Input: part model. Units: mm. Frame: model coordinates. A direction names the side the tool comes from. Coordinates: 2 decimals unless noted, no trailing zeros. Loops run counter-clockwise (first coordinate to the right, second up) from the corner with the lowest first, then second, coordinate; pieces in that order, holes last.
```python
from build123d import *

# Parameters (mm, degrees)
FACE003_W        = 10
FACE003_H        = 3
EXTRUDE003_DEPTH = 1
FACE002_W        = 10
FACE002_H        = 4
EXTRUDE002_DEPTH = 4
FACE001_W        = 8
FACE001_H        = 2.5
EXTRUDE001_DEPTH = 1.5
SKETCH_W         = 15
SKETCH_H         = 17
EXTRUDE_DEPTH    = 10
FACE004_W        = 29
FACE004_H        = 21
EXTRUDE004_DEPTH = 10


with BuildPart() as extrude003:
    # Face003 → Extrude003 (new body)
    with BuildSketch(Plane(origin=(7.5, 21, 2.5), x_dir=(1, 0, 0), z_dir=(0, 1, 0))):
        Rectangle(FACE003_W, FACE003_H)
    extrude(amount=EXTRUDE003_DEPTH)


with BuildPart() as fusion001:
    # Face002 → Extrude002 (new body)
    with BuildSketch(Plane(origin=(7.5, 17, 2), x_dir=(1, 0, 0), z_dir=(0, 1, 0))):
        Rectangle(FACE002_W, FACE002_H)
    extrude(amount=EXTRUDE002_DEPTH)

    # Fusion001: union Extrude003
    add(extrude003.part)


with BuildPart() as extrude001:
    # Face001 → Extrude001 (new body)
    with BuildSketch(Plane(origin=(7.624542, 0, 3.25), x_dir=(1, 0, 0), z_dir=(0, 1, 0))):
        Rectangle(FACE001_W, FACE001_H)
    extrude(amount=-EXTRUDE001_DEPTH)


with BuildPart() as fusion002:
    # Sketch → Extrude (new body)
    with BuildSketch(Plane.XY):
        with Locations((7.5, 8.5)):
            Rectangle(SKETCH_W, SKETCH_H)
    extrude(amount=EXTRUDE_DEPTH)

    # Fusion: union Extrude001
    add(extrude001.part)

    # Fusion002: union Fusion001
    add(fusion001.part)


with BuildPart() as cut:
    # Face004 → Extrude004 (new body)
    with BuildSketch(Plane(origin=(7.5, 10, 0), x_dir=(0, 1, 0), z_dir=(0, 0, 1))):
        Rectangle(FACE004_W, FACE004_H)
    extrude(amount=EXTRUDE004_DEPTH)

    # Cut: cut Fusion002
    add(fusion002.part, mode=Mode.SUBTRACT)


solid = cut.part
```
Item 1: Line query: L1, parallel to Y at x = 13, z = 5; L2, parallel to X at y = 13.5, z = 0.5; L3, parallel to Y at x = 8, z = 3.75. Output: solid intervals per line, ascending.
Result:
L1: y = -4.5 to 0, 17 to 24.5
L2: x = -3 to 0, 15 to 18
L3: y = -4.5 to -1.5, 22 to 24.5
Item 2: Section query A-A (z = 3.5). Output: boundary loops of the cut face in (x, y).
Result:
outline: (-3, -4.5) - (18, -4.5) - (18, 24.5) - (-3, 24.5) - close; hole (0, 0) - (3.62, 0) - (3.62, -1.5) - (11.62, -1.5) - (11.62, 0) - (15, 0) - (15, 17) - (12.5, 17) - (12.5, 22) - (2.5, 22) - (2.5, 17) - (0, 17) - close
Item 3: Mould query, pull axis X, two halves, no side actions, for faces 1 (the face through (7.4, 21.5, 1)), 2 (the face through (17, 10, 0)), 3 (the face through (7, 0, 5)), 4 (the face through (18, 10, 5)). Classes: +X half, -X half, draft (parallel to the pull), parting line (faces both ways), or undercut.
Result:
face 1: undercut
face 2: draft
face 3: undercut
face 4: +X half
Item 4: Reachability of faces 5 (the face through (7, 19, 10)), 6 (the face through (2.5, 19, 2)), 7 (the face through (15, 8, 5)) from +Z, -Z, +X, -X, +Y, -Y: full face, straight path, thin tool, end or side. Return the list, or none.
Result:
face 5: +Z, +X, -X, +Y, -Y
face 6: none
face 7: +Z, -Z
Item 5: Section query B-B (x = 8.25). Output: boundary loops of the cut face in (y, z).
Result:
outline: (-4.5, 0) - (0, 0) - (0, 2) - (-1.5, 2) - (-1.5, 4.5) - (0, 4.5) - (0, 10) - (-4.5, 10) - close; (17, 4) - (22, 4) - (22, 1) - (21, 1) - (21, 0) - (24.5, 0) - (24.5, 10) - (17, 10) - close
Item 6: Section query D-D (y = -0.5). Output: boundary loops of the cut face in (x, z), then the cut area to 3 significant figures.
Result:
outline: (-3, 0) - (18, 0) - (18, 10) - (-3, 10) - close; hole (3.62, 2) - (11.62, 2) - (11.62, 4.5) - (3.62, 4.5) - close
area: 190 mm2
Item 7: Section query C-C (y = 7.25). Output: boundary loops of the cut face in (x, z), then the cut area to 3 significant figures.
Result:
outline: (-3, 0) - (0, 0) - (0, 10) - (-3, 10) - close; (15, 0) - (18, 0) - (18, 10) - (15, 10) - close
area: 60.0 mm2
